```python
from build123d import *

# Parameters (mm, degrees)
F1_DEPTH = 120
F2_R     = 5
F3_DEPTH = 25
F4_R     = 5
F5_DEPTH = 25


with BuildPart() as f1:
    # F0 (on Top) → F1 (new body)
    with BuildSketch(Plane.XY):
        Polygon((-59, 0), (-86, 0), (-86, -2), (-61, -2), (-61, -62), (61, -62), (61, -2), (86, -2), (86, 0), (59, 0), (59, -60), (-59, -60), align=None)
    extrude(amount=F1_DEPTH)

    # F2 (on face) → F3 (cut)
    with BuildSketch(Plane.XZ.offset(2)):
        with Locations((-73.5, 97.5)):
            Circle(F2_R)
        with Locations((-73.5, 22.5)):
            Circle(F2_R)
    extrude(amount=-F3_DEPTH, mode=Mode.SUBTRACT)

    # F4 (on face) → F5 (cut)
    with BuildSketch(Plane.XZ.offset(2)):
        with Locations((72.881177, 97.5)):
            Circle(F4_R)
        with Locations((72.881177, 22.5)):
            Circle(F4_R)
    extrude(amount=-F5_DEPTH, mode=Mode.SUBTRACT)


solid = f1.part
```
CAD build for the part. Positions are in the model's coordinates, mm. A direction names the side the tool comes from. Give positions to 0.01 mm unless a question says otherwise; leave off trailing zeros. Write each loop counter-clockwise with the first axis right and the second up, starting at its lowest first coordinate (ties: lowest second). Pieces come first, ordered by that corner, then holes. Notation, with made-up numbers: M 2,46 L 28,46 A30 ccw 28,77 Z; hole C 18,28.5 d6. An arc over 180 degrees is marked long. Return JSON: item names as keys, results as strings. Group by question number.
(1) Drill centre lines: L1, parallel to X at y = -37.5, z = 78.5; L2, parallel to Y at x = 13, z = 11; L3, parallel to Y at x = 78, z = 111.5. Where is each one in solid material? Low to high. Write a range as [from, to].
(2) Flat gauge pins, fed straight in: pin 1 Ø20 at (x, z) = (-74.5, 77) entering from -Y; pin 2 Ø18 at (y, z) = (-20.5, 79) entering from +X; pin 3 Ø1 at (x, z) = (-15, 73) entering from +Y. Where does each tip first touch, or does it go through?
(3) 3-axis set-ups, long thin cutter, end or side, ignore diameter. For faces 1 (the face through (-74, -2, 59)), 2 (the face through (61, -32, 59)), 3 (the face through (73, 0, 59)), 4 (the face through (1, -60, 59)): which of +Z, -Z, +X, -X, +Y, -Y reach the whole face in a straight line?
(4) Band-saw the part on C-C (x = -73.5). Give the cut face in (y, z), and give its area (3 significant figures).
(5) Band-saw the part on D-D (z = 105). Give the cut face in (x, y).
(6) Mould opens along Z. For faces 5 (the face through (-61, -32, 59)), 6 (the face through (75.188, -1.014, 18.064)), 7 (the face through (0, -61, 120)) say: pulls with the +Z half, pulls with the -Z half, needs draft (parallel to the pull), parting line crosses it, or undercut.
(7) Band-saw the part on A-A (y = -25). Give the cut face in (x, z), and give its area (3 significant figures).
(8) Band-saw the part on B-B (z = 22.5). Give the cut face in (x, y).
Entries:
{
 "1": {"L1": "x = [-61, -59], [59, 61]", "L2": "y = [-62, -60]", "L3": "y = [-2, 0]"},
 "2": {"pin 1": "stops at y = -2", "pin 2": "stops at x = 61", "pin 3": "stops at y = -60"},
 "3": {"face 1": "+Z, -Z, -X, -Y", "face 2": "+Z, -Z, +X, -Y", "face 3": "+Z, -Z, +X, -X, +Y", "face 4": "+Z, -Z, +Y"},
 "4": {"outline": "M -2,0 L 0,0 L 0,17.5 L -2,17.5 Z; M -2,27.5 L 0,27.5 L 0,92.5 L -2,92.5 Z; M -2,102.5 L 0,102.5 L 0,120 L -2,120 Z", "area": "200 mm^2"},
 "5": {"outline": "M -86,-2 L -61,-2 L -61,-62 L 61,-62 L 61,-2 L 86,-2 L 86,0 L 59,0 L 59,-60 L -59,-60 L -59,0 L -86,0 Z"},
 "6": {"face 5": "needs draft", "face 6": "undercut", "face 7": "pulls with the +Z half"},
 "7": {"outline": "M -61,0 L -59,0 L -59,120 L -61,120 Z; M 59,0 L 61,0 L 61,120 L 59,120 Z", "area": "480 mm^2"},
 "8": {"outline": "M -86,-2 L -78.5,-2 L -78.5,0 L -86,0 Z; M -68.5,-2 L -61,-2 L -61,-62 L 61,-62 L 61,-2 L 67.88,-2 L 67.88,0 L 59,0 L 59,-60 L -59,-60 L -59,0 L -68.5,0 Z; M 77.88,-2 L 86,-2 L 86,0 L 77.88,0 Z"}
}
